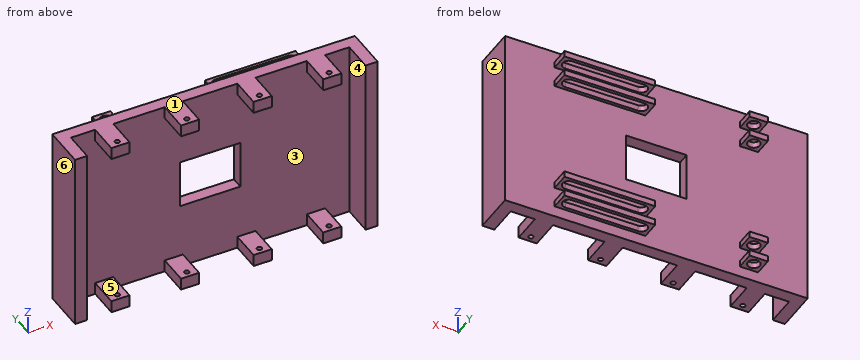
from build123d import *

# Parameters (mm, degrees)
SKETCH1_W               = 250
SKETCH1_H               = 150
SKETCH1_W_2             = 75
SKETCH1_H_2             = 5
SKETCH1_W_3             = 15
BOSS_EXTRUDE2_DEPTH     = 10
SKETCH1_8_W             = 75
SKETCH1_8_H             = 5
SKETCH1_8_W_2           = 15
BOSS_EXTRUDE3_DEPTH     = 25
SKETCH5_W               = 230
SKETCH5_H               = 130
BOSS_EXTRUDE4_DEPTH     = 25
SKETCH7_R               = 5
CUT_EXTRUDE2_DEPTH      = 120
CUT_EXTRUDE2_DEPTH_BACK = 32
CUT_EXTRUDE3_DEPTH      = 142
SKETCH9_W               = 50
SKETCH9_H               = 40
CUT_EXTRUDE4_DEPTH      = 10
SKETCH10_R              = 2
SKETCH10_W              = 42.5
SKETCH10_H              = 25
SKETCH10_W_2            = 20
SKETCH10_W_3            = 45
CUT_EXTRUDE5_DEPTH      = 1
CUT_EXTRUDE5_DEPTH_BACK = 151


with BuildPart() as part:
    # Sketch1 → Boss-Extrude2 (new body)
    with BuildSketch(Plane(origin=(0, 0, 0), x_dir=(1, 0, 0), z_dir=(0, 1, 0))):
        Rectangle(SKETCH1_W, SKETCH1_H)
        with Locations((46.5, -63.5)):
            Rectangle(SKETCH1_W_2, SKETCH1_H_2, mode=Mode.SUBTRACT)
        with Locations((-76.5, -63.5)):
            Rectangle(SKETCH1_W_3, SKETCH1_H_2, mode=Mode.SUBTRACT)
        with Locations((-76.5, -46.5)):
            Rectangle(SKETCH1_W_3, SKETCH1_H_2, mode=Mode.SUBTRACT)
        with Locations((46.5, -46.5)):
            Rectangle(SKETCH1_W_2, SKETCH1_H_2, mode=Mode.SUBTRACT)
        with Locations((46.5, 46.5)):
            Rectangle(SKETCH1_W_2, SKETCH1_H_2, mode=Mode.SUBTRACT)
        with Locations((46.5, 63.5)):
            Rectangle(SKETCH1_W_2, SKETCH1_H_2, mode=Mode.SUBTRACT)
        with Locations((-76.5, 63.5)):
            Rectangle(SKETCH1_W_3, SKETCH1_H_2, mode=Mode.SUBTRACT)
        with Locations((-76.5, 46.5)):
            Rectangle(SKETCH1_W_3, SKETCH1_H_2, mode=Mode.SUBTRACT)
    extrude(amount=BOSS_EXTRUDE2_DEPTH)

    # Sketch1<8> → Boss-Extrude3 (add)
    with BuildSketch(Plane(origin=(0, 0, 0), x_dir=(1, 0, 0), z_dir=(0, 1, 0))):
        with Locations((46.5, -63.5)):
            Rectangle(SKETCH1_8_W, SKETCH1_8_H)
        with Locations((-76.5, -63.5)):
            Rectangle(SKETCH1_8_W_2, SKETCH1_8_H)
        with Locations((-76.5, -46.5)):
            Rectangle(SKETCH1_8_W_2, SKETCH1_8_H)
        with Locations((46.5, -46.5)):
            Rectangle(SKETCH1_8_W, SKETCH1_8_H)
        with Locations((46.5, 46.5)):
            Rectangle(SKETCH1_8_W, SKETCH1_8_H)
        with Locations((46.5, 63.5)):
            Rectangle(SKETCH1_8_W, SKETCH1_8_H)
        with Locations((-76.5, 63.5)):
            Rectangle(SKETCH1_8_W_2, SKETCH1_8_H)
        with Locations((-76.5, 46.5)):
            Rectangle(SKETCH1_8_W_2, SKETCH1_8_H)
    extrude(amount=BOSS_EXTRUDE3_DEPTH)

    # Sketch5 → Boss-Extrude4 (add)
    with BuildSketch(Plane.XZ):
        Polygon((-125, 75), (-115, 75), (115, 75), (125, 75), (125, -75), (90, -75), (-90, -75), (-125, -75), align=None)
        Rectangle(SKETCH5_W, SKETCH5_H, mode=Mode.SUBTRACT)
    extrude(amount=BOSS_EXTRUDE4_DEPTH)

    # Sketch7 → Cut-Extrude2 (cut, two sides)
    with BuildSketch(Plane(origin=(0, 0, 44), x_dir=(-1, 0, 0), z_dir=(0, 0, -1))) as cut_extrude2_sk:
        with Locations((76.5, 17.5)):
            Circle(SKETCH7_R)
    extrude(amount=CUT_EXTRUDE2_DEPTH, mode=Mode.SUBTRACT)
    extrude(cut_extrude2_sk.sketch, amount=-CUT_EXTRUDE2_DEPTH_BACK, mode=Mode.SUBTRACT)

    # Sketch8 → Cut-Extrude3 (cut, through all)
    with BuildSketch(Plane.XY.offset(66)):
        with BuildLine():
            Line((16.5, 22.5), (76.5, 22.5))
            ThreePointArc((76.5, 22.5), (81.5, 17.5), (76.5, 12.5))
            Line((76.5, 12.5), (16.5, 12.5))
            ThreePointArc((16.5, 12.5), (11.5, 17.5), (16.5, 22.5))
        make_face()
    extrude(amount=-CUT_EXTRUDE3_DEPTH, mode=Mode.SUBTRACT)

    # Sketch9 → Cut-Extrude4 (cut)
    with BuildSketch(Plane(origin=(0, 10, 0), x_dir=(1, 0, 0), z_dir=(0, 1, 0))):
        Rectangle(SKETCH9_W, SKETCH9_H)
    extrude(amount=-CUT_EXTRUDE4_DEPTH, mode=Mode.SUBTRACT)

    # Sketch10 → Cut-Extrude5 (cut, two sides)
    with BuildSketch(Plane.XY.offset(75)) as cut_extrude5_sk:
        with Locations((-87.5, -20)):
            Circle(SKETCH10_R)
        with Locations((87.5, -20)):
            Circle(SKETCH10_R)
        with Locations((-30, -20)):
            Circle(SKETCH10_R)
        with Locations((30, -20)):
            Circle(SKETCH10_R)
        with Locations((-58.75, -12.5)):
            Rectangle(SKETCH10_W, SKETCH10_H)
        with Locations((-105, -12.5)):
            Rectangle(SKETCH10_W_2, SKETCH10_H)
        with Locations((0, -12.5)):
            Rectangle(SKETCH10_W_3, SKETCH10_H)
        with Locations((58.75, -12.5)):
            Rectangle(SKETCH10_W, SKETCH10_H)
        with Locations((105, -12.5)):
            Rectangle(SKETCH10_W_2, SKETCH10_H)
    extrude(amount=CUT_EXTRUDE5_DEPTH, mode=Mode.SUBTRACT)
    extrude(cut_extrude5_sk.sketch, amount=-CUT_EXTRUDE5_DEPTH_BACK, mode=Mode.SUBTRACT)


solid = part.part
Here's how the part is built. I have some questions about the finished solid (model axes, mm). Face numbers are marked on the shaded views. A direction names the side the tool comes from. Coordinates: 2 decimals unless noted, no trailing zeros. Write each loop counter-clockwise with the first axis right and the second up, starting at its lowest first coordinate (ties: lowest second). Pieces come first, ordered by that corner, then holes. Notation, with made-up numbers: (34.25, 1) - (83.25, 1) arc R17 cw to (83.25, 19) - close; hole circle Ø3 at (-36.75, 23.25). An arc over 180 degrees is marked (long way). Use one line per item in the form item = value.
1) Suppose I cut it at A-A, the plane x = 0.5. Write out the boundary of the cut face in (y, z), plus the area to 3 significant figures.
Solved:
outline = (0, -75) - (10, -75) - (10, -20) - (0, -20) - close; (0, 20) - (10, 20) - (10, 75) - (0, 75) - close
area = 1,100 mm2
2) Suppose I cut it at C-C, the plane y = 6.5. Write out the boundary of the cut face in (x, z), plus the area to 3 significant figures.
Solved:
outline = (-125, -75) - (125, -75) - (125, 75) - (-125, 75) - close; hole (-25, -20) - (25, -20) - (25, 20) - (-25, 20) - close
area = 35,500 mm2
3) On a 3-axis mill with a long thin cutter (end or side, diameter ignored), from which of +Z, -Z, +X, -X, +Y, -Y can I reach the whole of each face in a straight line? I mean the marked faces 5 and 6. Say none if no direction works.
Solved:
face_5 = -Y
face_6 = +Z, -Z, -X, +Y, -Y
4) I need wall thicknesses on line 1 (Z direction, x = -71, y = 14.5); line 2 (Y direction, x = -76, z = -64); line 3 (X direction, y = -8.5, z = 37.5). Which ranges of each line are inside material? Lowest first, please.
Solved:
line_1 = -66 to -61, -49 to -44, 44 to 49, 61 to 66
line_2 = 0 to 12.53, 22.47 to 25
line_3 = -125 to -115, 115 to 125
5) Suppose I cut it at B-B, the plane z = 25. Write out the boundary of the cut face in (x, y).
Solved:
outline = (-125, -25) - (-115, -25) - (-115, 0) - (115, 0) - (115, -25) - (125, -25) - (125, 10) - (-125, 10) - close
6) Suppose I cut it at D-D, the plane y = -4. Give the number of separate pieces and of enclosed holes in the cut face, plus the area to 3 significant figures.
Solved:
separate_pieces = 10
enclosed_holes = 0
area = 4,200 mm2
7) I'm going to push flat-ended pins straight in: P1, Ø16, axis at x = -76.5, y = 17.5, coming from the +Z side; P2, Ø12, axis at x = -49.5, z = 37.5, coming from the +Y side; P3, Ø1.5, axis at y = 19, z = 64, coming from the +X side; P4, Ø16.5, axis at x = 44.5, y = 20.5, coming from the -Z side. Where does each tip first touch, or does it pass through?
Solved:
P1 = 75
P2 = 10
P3 = 84
P4 = -66
8) Thinking about a two-plate mould opening in X: for the marked faces 1, 2, 3 and 4, which applies, released by +X, released by -X, zero draft, split by the parting line, or undercut?
Solved:
face_1 = zero draft
face_2 = released by +X
face_3 = undercut
face_4 = undercut
